The listing builds one solid part. Answer for the finished solid, in the listing's coordinates (mm). Give positions to 0.01 mm unless a question says otherwise; leave off trailing zeros. Write each loop counter-clockwise with the first axis right and the second up, starting at its lowest first coordinate (ties: lowest second). Pieces come first, ordered by that corner, then holes. Notation, with made-up numbers: M 53,-6.75 L 100,-6.75 A18 cw 100,26.25 Z; hole C 1,56 d10. An arc over 180 degrees is marked long. Return JSON: item names as keys, results as strings.
Solid Edge part; units mm, degrees
sketch "Sketch1" plane through (0, 0, 0) normal (1, 0, 0) x (0, 1, 0)
  line L0 (-105.6532, 103.7678) -> (-70.6532, 103.7678)
  line L1 (-70.6532, 103.7678) -> (-70.6532, 98.7678)
  line L2 (-70.6532, 98.7678) -> (-60.6532, 98.7678)
  line L3 (-60.6532, 98.7678) -> (-60.6532, 103.7678)
  line L4 (-60.6532, 103.7678) -> (69.3468, 103.7678)
  line L5 (69.3468, 103.7678) -> (69.3468, 98.7678)
  line L6 (69.3468, 98.7678) -> (79.3468, 98.7678)
  line L7 (79.3468, 98.7678) -> (79.3468, 103.7678)
  line L8 (79.3468, 103.7678) -> (94.3468, 103.7678)
  line L9 (94.3468, 103.7678) -> (94.3468, 78.7678)
  line L10 (94.3468, 78.7678) -> (91.3468, 78.7678)
  line L11 (91.3468, 78.7678) -> (91.3468, 28.7678)
  line L12 (91.3468, 28.7678) -> (94.3468, 28.7678)
  line L13 (94.3468, 28.7678) -> (94.3468, 3.7678)
  line L14 (94.3468, 3.7678) -> (44.3468, 3.7678)
  line L15 (44.3468, 3.7678) -> (44.3468, 6.7678)
  line L16 (44.3468, 6.7678) -> (-55.6532, 6.7678)
  line L17 (-55.6532, 6.7678) -> (-55.6532, 3.7678)
  line L18 (-55.6532, 3.7678) -> (-105.6532, 3.7678)
  line L19 (-105.6532, 3.7678) -> (-105.6532, 28.7678)
  line L20 (-105.6532, 28.7678) -> (-102.6532, 28.7678)
  line L21 (-102.6532, 28.7678) -> (-102.6532, 78.7678)
  line L22 (-102.6532, 78.7678) -> (-105.6532, 78.7678)
  line L23 (-105.6532, 78.7678) -> (-105.6532, 103.7678)
  dimension "D1" = 70.6532
  dimension "D2" = 44.3468
  dimension "D3" = 91.3468
  dimension "D4" = 94.3468
  dimension "D5" = 69.3468
  dimension "D6" = 44.3468
  dimension "D7" = 70.6532
extrude "Protrusion1" add sketch "Sketch1" against normal blind 3
properties material "Acier"
Item 1: Given pin 1 Ø1.5 at (x, z) = (-1, 59) entering from -Y; pin 2 Ø0.9 at (x, y) = (-1, -65) entering from +Z, each flat-ended and moving along its own axis, determine where each tip first touches the part or whether it passes through.
Geometry results:
{"pin 1": "stops at y = -102.65", "pin 2": "stops at z = 98.77"}
Item 2: A cutting plane is placed at B-B, the plane y = -28. Write down the section's boundary in (x, z).
Geometry results:
{"outline": "M -3,6.77 L 0,6.77 L 0,103.77 L -3,103.77 Z"}
Item 3: A cutting plane is placed at C-C, the plane z = 50.5. Write down the section's boundary in (x, y), plus the area to 3 significant figures.
Geometry results:
{"outline": "M -3,-102.65 L 0,-102.65 L 0,91.35 L -3,91.35 Z", "area": "582 mm2"}
Item 4: Find the intervals of material crossed by line 1 (Z direction, x = -2.65, y = -0.5); line 2 (Y direction, x = -0.85, z = 40); line 3 (Z direction, x = -0.3, y = -67), in increasing order.
Geometry results:
{"line 1": "z = 6.77 to 103.77", "line 2": "y = -102.65 to 91.35", "line 3": "z = 3.77 to 98.77"}
Item 5: A cutting plane is placed at A-A, the plane x = -1.9. Write down the section's boundary in (y, z), plus the area to 3 significant figures.
Geometry results:
{"outline": "M -105.65,3.77 L -55.65,3.77 L -55.65,6.77 L 44.35,6.77 L 44.35,3.77 L 94.35,3.77 L 94.35,28.77 L 91.35,28.77 L 91.35,78.77 L 94.35,78.77 L 94.35,103.77 L 79.35,103.77 L 79.35,98.77 L 69.35,98.77 L 69.35,103.77 L -60.65,103.77 L -60.65,98.77 L -70.65,98.77 L -70.65,103.77 L -105.65,103.77 L -105.65,78.77 L -102.65,78.77 L -102.65,28.77 L -105.65,28.77 Z", "area": "19,300 mm2"}
